Design review of the part shown in the three views and the two pictorial views. Dimensions are in mm from the part's minimum x, y and z. A direction names the side the tool comes from. Coordinates: 2 decimals unless noted, no trailing zeros. Write each loop counter-clockwise with the first axis right and the second up, starting at its lowest first coordinate (ties: lowest second). Pieces come first, ordered by that corner, then holes. Notation, with made-up numbers: M -19,5.25 L 39,5.25 A25 cw 39,26.25 Z; hole C 80.5,63 d3. An arc over 180 degrees is marked long. One line per question, with ' | ' between items.
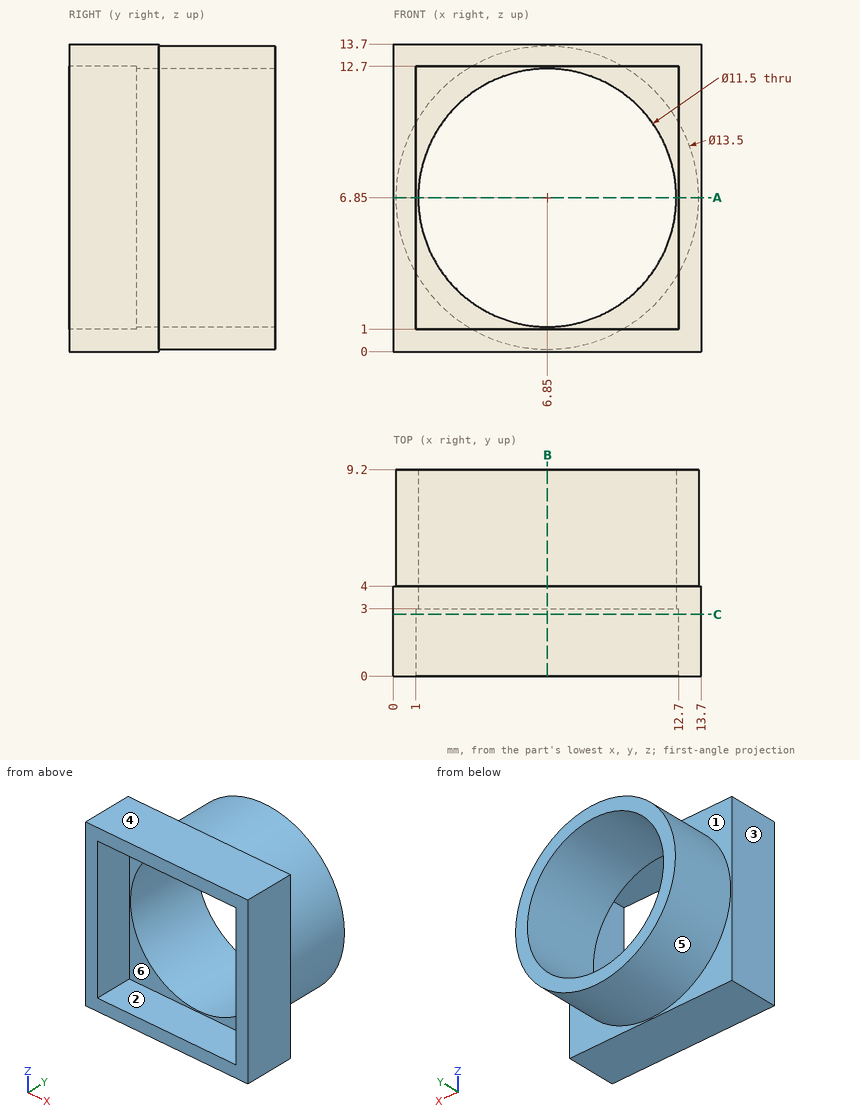
1. Draft analysis for pull direction Z (two halves, no side actions). For the marked faces 4, 5 and 6, state which applies: pulls with the +Z half, pulls with the -Z half, needs draft (parallel to the pull), parting line crosses it, or undercut.
Computed values:
face 4: pulls with the +Z half | face 5: parting line crosses it | face 6: undercut
2. Take a section at A-A on z = 6.85. State the section outline as (x, y) points.
Computed values:
outline: M 0,0 L 1,0 L 1,3 L 1.1,3 L 1.1,9.2 L 0.1,9.2 L 0.1,4 L 0,4 Z; M 12.6,3 L 12.7,3 L 12.7,0 L 13.7,0 L 13.7,4 L 13.6,4 L 13.6,9.2 L 12.6,9.2 Z
3. Machinability: for the marked faces 1, 2 and 3, which of the approach directions +Z, -Z, +X, -X, +Y, -Y give a long, thin tool a straight path to every point of the face, cutting with its end or side? Answer none if there is none.
Computed values:
face 1: +Y | face 2: -Y | face 3: +Z, -Z, -X, +Y, -Y
4. Take a section at B-B on x = 6.85. State the section outline as (y, z) points, plus the area to 3 significant figures.
Computed values:
outline: M 0,0 L 4,0 L 4,0.1 L 9.2,0.1 L 9.2,1.1 L 3,1.1 L 3,1 L 0,1 Z; M 0,12.7 L 3,12.7 L 3,12.6 L 9.2,12.6 L 9.2,13.6 L 4,13.6 L 4,13.7 L 0,13.7 Z | area: 18.6 mm2
5. For line 1 along X through (y, z) = (7, 6.85); line 2 along X through (y, z) = (1.25, 2.5), list the stretches that pass through material, from the lowest coordinate up.
Computed values:
line 1: x = 0.1 to 1.1, 12.6 to 13.6 | line 2: x = 0 to 1, 12.7 to 13.7
6. Take a section at C-C on y = 2.75. State the section outline as (x, z) points.
Computed values:
outline: M 0,0 L 13.7,0 L 13.7,13.7 L 0,13.7 Z; hole M 1,1 L 12.7,1 L 12.7,12.7 L 1,12.7 Z
7. Clearance check with flat-ended pins moving along their axes: P1, Ø2, axis at y = 7, z = 11, coming from the +X side; P2, Ø1.5, axis at x = 3.5, z = 11, coming from the +Y side; P3, Ø3, axis at y = 7.5, z = 11.5, coming from the -X side. State where each tip first meets the part, or that it passes through.
Computed values:
P1: stops at x = 12.82 | P2: stops at y = 9.2 | P3: stops at x = 0.88
